from build123d import *

# Parameters (mm, degrees)
MOUNTING_DEPTH          = 3
SKETCH3_R               = 1.5
BOSS_EXTRUDE2_DEPTH     = 6
PIVOTHOLE_DEPTH         = 133.681535985
PIVOTHOLE_DEPTH_BACK    = 133.681535985
SKETCH3_2_R             = 1.5
SKETCH4_W               = 6
SKETCH4_H               = 12.7
TAB_DEPTH               = 6
FILLET1_R               = 12.7
FILLET2_R               = 2.54
TABFILLET_R             = 1.27
CUT_EXTRUDE2_DEPTH      = 133.681535985
CUT_EXTRUDE2_DEPTH_BACK = 133.681535985
SKETCH5_W               = 12.954
SKETCH5_H               = 6


with BuildPart() as part:
    # Sketch2 → Mounting (new, symmetric)
    with BuildSketch(Plane(origin=(0, 0, 0), x_dir=(0, 0, -1), z_dir=(1, 0, 0))):
        Polygon((-60.325, -47.8), (-60.325, -9.7), (60.325, -9.7), (60.325, -47.8), (57.15, -47.8), (44.45, -47.8), (41.275, -47.8), (41.275, -41.45), (-41.275, -41.45), (-41.275, -47.8), (-44.45, -47.8), (-57.15, -47.8), align=None)
    extrude(amount=MOUNTING_DEPTH, both=True)

    # Sketch3 → Boss-Extrude2 (add)
    # profile 1 of 2: a face of its own
    with BuildSketch(Plane(origin=(3, 0, 0), x_dir=(0, 0, -1), z_dir=(1, 0, 0))):
        with Locations((41.275, -35.1)):
            Circle(SKETCH3_R)
    # profile 2 of 2: a face of its own
    with BuildSketch(Plane(origin=(3, 0, 0), x_dir=(0, 0, -1), z_dir=(1, 0, 0))):
        with BuildLine():
            Line((64.196478559, 68.417190639), (-60.325, -9.7))
            Line((-60.325, -9.7), (60.325, -9.7))
            Line((60.325, -9.7), (104.734943372, 30.73838178))
            ThreePointArc((104.734943372, 30.73838178), (105.039779736, 31.035237071), (105.324051376, 31.351840779))
            Line((105.324051376, 31.351840779), (111.446603358, 38.648414099))
            ThreePointArc((111.446603358, 38.648414099), (112.908057477, 43.283554387), (110.663922466, 47.594497635))
            ThreePointArc((110.663922466, 47.594497635), (91.120762799, 60.652819442), (69.214515919, 69.171692948))
            ThreePointArc((69.214515919, 69.171692948), (66.626854298, 69.317479577), (64.196478559, 68.417190639))
        make_face()
        with BuildLine():
            ThreePointArc((107.546402559, 43.879182086), (88.881282025, 56.350816901), (67.95924355, 64.48695269))
            ThreePointArc((67.95924355, 64.48695269), (66.122126243, 63.426292519), (67.182786415, 61.589175212))
            ThreePointArc((67.182786415, 61.589175212), (87.496036185, 53.689784401), (105.61803973, 41.581048756))
            ThreePointArc((105.61803973, 41.581048756), (107.731287809, 41.765934006), (107.546402559, 43.879182086))
        make_face(mode=Mode.SUBTRACT)
        with BuildLine():
            ThreePointArc((101.423850576, 36.582608765), (84.483126483, 47.902038715), (65.493992145, 55.286509195))
            ThreePointArc((65.493992145, 55.286509195), (63.656874838, 54.225849023), (64.71753501, 52.388731716))
            ThreePointArc((64.71753501, 52.388731716), (83.097880644, 45.241006215), (99.495487747, 34.284475436))
            ThreePointArc((99.495487747, 34.284475436), (101.608735827, 34.469360686), (101.423850576, 36.582608765))
        make_face(mode=Mode.SUBTRACT)
    extrude(amount=-BOSS_EXTRUDE2_DEPTH)

    # Sketch3<2> → PivotHole (cut, two sides: drawn at the far end of the back side and taken through both)
    with BuildSketch(Plane(origin=(3, 0, 0), x_dir=(0, 0, -1), z_dir=(1, 0, 0)).offset(-PIVOTHOLE_DEPTH_BACK)):
        with Locations((41.275, -35.1)):
            Circle(SKETCH3_2_R)
    extrude(amount=PIVOTHOLE_DEPTH + PIVOTHOLE_DEPTH_BACK, mode=Mode.SUBTRACT)

    # Sketch4 → Tab (add)
    with BuildSketch(Plane.XZ.offset(47.8)):
        with Locations((0, 50.8)):
            Rectangle(SKETCH4_W, SKETCH4_H)
        with Locations((0, -50.8)):
            Rectangle(SKETCH4_W, SKETCH4_H)
    extrude(amount=TAB_DEPTH)

    # Fillet1
    fillet1_edges = [part.edges().sort_by_distance(p)[0] for p in [
        (0, -9.7, 60.325),
        (0, -9.7, -60.325),
    ]]
    fillet(fillet1_edges, radius=FILLET1_R)

    # Fillet2
    fillet2_edges = [part.edges().sort_by_distance(p)[0] for p in [
        (0, -47.8, 60.325),
        (0, -47.8, -60.325),
        (0, -47.8, -41.275),
        (0, -41.45, -41.275),
        (0, -41.45, 41.275),
        (0, -47.8, 41.275),
    ]]
    fillet(fillet2_edges, radius=FILLET2_R)

    # TabFillet
    tabfillet_edges = [part.edges().sort_by_distance(p)[0] for p in [
        (0, -53.8, 57.15),
        (0, -53.8, 44.45),
        (0, -53.8, -44.45),
        (0, -53.8, -57.15),
    ]]
    fillet(tabfillet_edges, radius=TABFILLET_R)

    # Sketch5 → Cut-Extrude2 (cut, two sides: drawn at the far end of the back side and taken through both)
    with BuildSketch(Plane(origin=(3, 0, 0), x_dir=(0, 0, -1), z_dir=(1, 0, 0)).offset(-CUT_EXTRUDE2_DEPTH_BACK)):
        with Locations((-88.9, -25.4)):
            Rectangle(SKETCH5_W, SKETCH5_H)
        with Locations((-63.5, -25.4)):
            Rectangle(SKETCH5_W, SKETCH5_H)
        with Locations((-38.1, -25.4)):
            Rectangle(SKETCH5_W, SKETCH5_H)
        with Locations((-12.7, -25.4)):
            Rectangle(SKETCH5_W, SKETCH5_H)
        with Locations((12.7, -25.4)):
            Rectangle(SKETCH5_W, SKETCH5_H)
        with Locations((38.1, -25.4)):
            Rectangle(SKETCH5_W, SKETCH5_H)
        with Locations((63.5, -25.4)):
            Rectangle(SKETCH5_W, SKETCH5_H)
        with Locations((88.9, -25.4)):
            Rectangle(SKETCH5_W, SKETCH5_H)
    extrude(amount=CUT_EXTRUDE2_DEPTH + CUT_EXTRUDE2_DEPTH_BACK, mode=Mode.SUBTRACT)


solid = part.part
Read the model definition and answer for the solid it produces. Units are mm, in the model's axes. A direction names the side the tool comes from. Give positions to 0.01 mm unless a question says otherwise; leave off trailing zeros. Write each loop counter-clockwise with the first axis right and the second up, starting at its lowest first coordinate (ties: lowest second). Pieces come first, ordered by that corner, then holes. Notation, with made-up numbers: (39, 34.5) - (77, 34.5) arc R14 cw to (77, 47.5) - close; hole circle Ø8 at (-22.5, 67). An arc over 180 degrees is marked (long way). Answer in a Markdown table with one row per item. Add a question column.
Item 1: Section C-C, the plane z = -96 is taken. Write down the section's boundary in (x, y), and give its area (3 significant figures).
Item 2: A tool of negligible diameter and unlimited length cuts with its end or side. For faces 1 (the face through (0, -50, -44.45)), 2 (the face through (0, -25, -57.023)), 3 (the face through (-0.04, -10.11, -61.44)), 4 (the face through (0, -25, -19.177)), from which of +Z, -Z, +X, -X, +Y, -Y can it reach the whole face along a straight path? Write none if from no direction.
Item 3: Section A-A, the plane z = -78 is taken. Write down the section's boundary in (x, y), and give its area (3 significant figures).
Item 4: Find the intervals of material crossed by L1, parallel to Y at x = 1.95, z = -91; L2, parallel to Z at x = -0.25, y = -35.1 (3 decimals); L3, parallel to Y at x = 0.75, z = -73, in increasing order.
Item 5: Flat-ended cylindrical pins translate along their axes: P1, Ø0.7, axis at x = -1.5, z = 44, coming from the -Y side; P2, Ø2, axis at x = -1, z = -94.5, coming from the -Y side; P3, Ø1.4, axis at x = 0.5, y = -44.5, coming from the -Z side (3 decimals). Find the tip coordinate at first contact, or state that the pin passes through.
Item 6: Section B-B, the plane x = -0.25 is taken. Count the separate pieces of the cut face and the enclosed holes in it, and give its area (3 significant figures).
Item 7: Determine the mould class of faces 5 (the face through (0, -50, 57.15)), 6 (the face through (0, -25, -31.623)), 7 (the face through (0, -22.4, -59)), 8 (the face through (0.042, 69.323, -66.663)) for opening direction Z: pulls with the +Z half, pulls with the -Z half, needs draft (parallel to the pull), parting line crosses it, or undercut.
Recorded:
| question | item | result |
|---|---|---|
| 1 | outline | (-3, 22.78) - (3, 22.78) - (3, 37.07) - (-3, 37.07) - close; (-3, 40.8) - (3, 40.8) - (3, 48.72) - (-3, 48.72) - close; (-3, 52.28) - (3, 52.28) - (3, 57.95) - (-3, 57.95) - close |
| 1 | area | 167 mm2 |
| 2 | face 1 | +X, -X, -Y |
| 2 | face 2 | -Z, +X, -X |
| 2 | face 3 | -Z, +X, -X, -Y |
| 2 | face 4 | +X, -X |
| 3 | outline | (-3, 6.39) - (3, 6.39) - (3, 47.7) - (-3, 47.7) - close; (-3, 50.97) - (3, 50.97) - (3, 58.02) - (-3, 58.02) - close; (-3, 61.24) - (3, 61.24) - (3, 66.41) - (-3, 66.41) - close |
| 3 | area | 321 mm2 |
| 4 | L1 | y = 18.23 to 40.61, 44.17 to 51.78, 55.22 to 60.72 |
| 4 | L2 | z = -60.325 to -42.775, -39.775 to 60.325 |
| 4 | L3 | y = 1.84 to 49.74, 52.93 to 59.84, 63 to 68.08 |
| 5 | P1 | stops at y = -47.8 |
| 5 | P2 | stops at y = 20.51 |
| 5 | P3 | stops at z = -60.325 |
| 6 | separate pieces | 1 |
| 6 | enclosed holes | 7 |
| 6 | area | 10,600 mm2 |
| 7 | face 5 | pulls with the +Z half |
| 7 | face 6 | undercut |
| 7 | face 7 | needs draft |
| 7 | face 8 | parting line crosses it |
